Source: CAD feature listing. Evaluate the final solid. Frame: model axes, mm. Face numbers are marked on the shaded views. A direction names the side the tool comes from. Give positions to 0.01 mm unless a question says otherwise; leave off trailing zeros. Order: outer loops, then holes, each group sorted by start corner. A loop starts at its lowest first (then second) coordinate and runs counter-clockwise, first axis right, second up. Notation, with made-up numbers: M 46,32 L 82,32 A22 ccw 82,50 Z; hole C -32.5,82.5 d9. An arc over 180 degrees is marked long. Answer in a Markdown table with one row per item. Add a question column.
(1) Section query B-B, the plane x = -9. Return loops of the section in (y, z), plus the area to 3 significant figures.
(2) Pin query (flat end, axial travel): P1, Ø6.5, axis at x = -16, z = -5.5, coming from the +Y side; P2, Ø2.5, axis at x = -28, z = -14, coming from the +Y side; P3, Ø1.5, axis at x = -34, z = 20.5, coming from the +Y side. Return the tip coordinate at first contact, or that it passes through.
(3) Mould query, pull axis Z, two halves, no side actions, for the marked faces 1, 2, 3 and 4. Classes: pulls with the +Z half, pulls with the -Z half, needs draft (parallel to the pull), parting line crosses it, or undercut.
(4) Section query C-C, the plane z = -16.5. Return loops of the section in (x, y), plus the area to 4 significant figures.
(5) Material intervals for line 1 along X through (y, z) = (26.5, -16); line 2 along X through (y, z) = (27.5, -20); line 3 along X through (y, z) = (19.5, -5), sorted ascending.
(6) Set-up query: the marked faces 5, 6 and 7. Return all of +Z, -Z, +X, -X, +Y, -Y with unobstructed straight access to the full face (end or side cutting, diameter ignored); none if empty.
(7) Section query D-D, the plane z = 13.5. Return loops of the section in (x, y), plus the area to 4 significant figures.
(8) Section query A-A, the plane y = 19.5. Return loops of the section in (x, z).
from build123d import *

# Parameters (mm, degrees)
SKETCH_1_W          = 47.5
SKETCH_1_H          = 60.8
EXTRUDE_1_DEPTH     = 30
SKETCH_2_R          = 1
EXTRUDE_3_DEPTH     = 5
SKETCH_3_W          = 37.5
SKETCH_3_H          = 45.8
CUT_EXTRUDE_1_DEPTH = 27
SKETCH_4_W          = 14
SKETCH_4_H          = 5
CUT_EXTRUDE_2_DEPTH = 8
SKETCH_5_R          = 3
SKETCH_5_W          = 6
SKETCH_5_H          = 6
EXTRUDE_4_DEPTH     = 20.5
SKETCH_6_W          = 5
SKETCH_6_H          = 10.5
EXTRUDE_6_DEPTH     = 25
SKETCH_7_R          = 1
EXTRUDE_7_DEPTH     = 5
SKETCH_12_W         = 5.3
SKETCH_12_H         = 4.5
CUT_EXTRUDE_5_DEPTH = 10
SKETCH_13_W         = 1.5
SKETCH_13_H         = 6
EXTRUDE_8_DEPTH     = 4.5


with BuildPart() as part:
    # 草图1 → 凸台-拉伸1 (new body)
    with BuildSketch(Plane(origin=(0, 0, 0), x_dir=(1, 0, 0), z_dir=(0, 1, 0))):
        with Locations((-26.283333333, -1.583333333)):
            Rectangle(SKETCH_1_W, SKETCH_1_H)
    extrude(amount=EXTRUDE_1_DEPTH)

    # 草图2 → 凸台-拉伸3 (add)
    with BuildSketch(Plane(origin=(0, 30, 0), x_dir=(1, 0, 0), z_dir=(0, 1, 0))):
        with Locations(Location((-22.533333333, 26.316666667, 0), (0, 0, 270))):
            Circle(SKETCH_2_R)
        with Locations(Location((-47.533333333, 26.316666667, 0), (0, 0, 270))):
            Circle(SKETCH_2_R)
        with Locations(Location((-47.533333333, -29.483333333, 0), (0, 0, 270))):
            Circle(SKETCH_2_R)
        with Locations(Location((-5.033333333, -29.483333333, 0), (0, 0, 270))):
            Circle(SKETCH_2_R)
    extrude(amount=EXTRUDE_3_DEPTH)

    # 草图3 → 切除-拉伸1 (cut)
    with BuildSketch(Plane(origin=(0, 30, 0), x_dir=(1, 0, 0), z_dir=(0, 1, 0))):
        with Locations((-26.283333333, -4.083333333)):
            Rectangle(SKETCH_3_W, SKETCH_3_H)
    extrude(amount=-CUT_EXTRUDE_1_DEPTH, mode=Mode.SUBTRACT)

    # 草图4 → 切除-拉伸2 (cut)
    with BuildSketch(Plane(origin=(0, 30, 0), x_dir=(1, 0, 0), z_dir=(0, 1, 0))):
        with Locations((-26.083333333, -29.483333333)):
            Rectangle(SKETCH_4_W, SKETCH_4_H)
    extrude(amount=-CUT_EXTRUDE_2_DEPTH, mode=Mode.SUBTRACT)

    # 草图5 → 凸台-拉伸4 (add)
    with BuildSketch(Plane(origin=(0, 3, 0), x_dir=(1, 0, 0), z_dir=(0, 1, 0))):
        with Locations(Location((-16.083333333, 4.816666667, 0), (0, 0, 270))):
            Circle(SKETCH_5_R)
        with Locations(Location((-36.483333333, 4.816666667, 0), (0, 0, 270))):
            Circle(SKETCH_5_R)
        with Locations((-25.533333333, -23.983333333)):
            Rectangle(SKETCH_5_W, SKETCH_5_H)
    extrude(amount=EXTRUDE_4_DEPTH)

    # 草图6 → 凸台-拉伸6 (add)
    with BuildSketch(Plane(origin=(0, 3, 0), x_dir=(1, 0, 0), z_dir=(0, 1, 0))):
        with Locations((-28.533333333, 13.566666667)):
            Rectangle(SKETCH_6_W, SKETCH_6_H)
    extrude(amount=EXTRUDE_6_DEPTH)

    # 草图7 → 凸台-拉伸7 (add)
    with BuildSketch(Plane(origin=(0, 23.5, 0), x_dir=(1, 0, 0), z_dir=(0, 1, 0))):
        with Locations(Location((-36.483333333, 4.816666667, 0), (0, 0, 270))):
            Circle(SKETCH_7_R)
        with Locations(Location((-16.083333333, 4.816666667, 0), (0, 0, 270))):
            Circle(SKETCH_7_R)
    extrude(amount=EXTRUDE_7_DEPTH)

    # 草图12 → 切除-拉伸5 (cut)
    with BuildSketch(Plane(origin=(0, 0, -28.816666667), x_dir=(-1, 0, 0), z_dir=(0, 0, -1))):
        with Locations((13.183333333, 27.75)):
            Rectangle(SKETCH_12_W, SKETCH_12_H)
    extrude(amount=-CUT_EXTRUDE_5_DEPTH, mode=Mode.SUBTRACT)

    # 草图13 → 凸台-拉伸8 (add)
    with BuildSketch(Plane(origin=(0, 25.5, 0), x_dir=(1, 0, 0), z_dir=(0, 1, 0))):
        with Locations((-13.183333333, 21.816666667)):
            Rectangle(SKETCH_13_W, SKETCH_13_H)
    extrude(amount=EXTRUDE_8_DEPTH)


solid = part.part
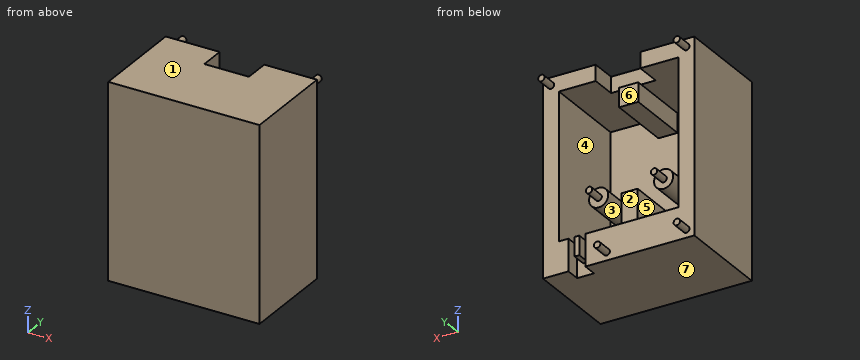
Values follow:
| question | item | result |
|---|---|---|
| 1 | outline | M 0,-28.82 L 30,-28.82 L 30,-18.82 L 3,-18.82 L 3,26.98 L 30,26.98 L 30,31.98 L 0,31.98 Z |
| 1 | area | 587 mm² |
| 2 | P1 | stops at y = 28.5 |
| 2 | P2 | stops at y = 28 |
| 2 | P3 | stops at y = 3 |
| 3 | face 1 | pulls with the +Z half |
| 3 | face 2 | needs draft |
| 3 | face 3 | undercut |
| 3 | face 4 | undercut |
| 4 | outline | M -50.03,0 L -2.53,0 L -2.53,30 L -7.53,30 L -7.53,3 L -26.03,3 L -26.03,28 L -31.03,28 L -31.03,3 L -45.03,3 L -45.03,30 L -50.03,30 Z |
| 4 | area | 537.5 mm² |
| 5 | line 1 | x = -50.03 to -45.03, -31.03 to -26.03, -7.53 to -2.53 |
| 5 | line 2 | x = -50.03 to -15.83, -13.93 to -12.43, -10.53 to -2.53 |
| 5 | line 3 | x = -50.03 to -45.03, -39.48 to -33.49, -19.08 to -13.09, -7.53 to -2.53 |
| 6 | face 5 | +Y |
| 6 | face 6 | +Z, +Y |
| 6 | face 7 | -Z, +X, -X, +Y, -Y |
| 7 | outline | M -50.03,0 L -2.53,0 L -2.53,30 L -7.53,30 L -7.53,3 L -45.03,3 L -45.03,30 L -50.03,30 Z |
| 7 | area | 412.5 mm² |
| 8 | outline | M -50.03,-28.82 L -2.53,-28.82 L -2.53,31.98 L -50.03,31.98 Z; C -36.48,-4.82 d6; C -16.08,-4.82 d6; hole M -45.03,-18.82 L -31.03,-18.82 L -31.03,-8.32 L -26.03,-8.32 L -26.03,-18.82 L -7.53,-18.82 L -7.53,26.98 L -22.53,26.98 L -22.53,20.98 L -28.53,20.98 L -28.53,26.98 L -45.03,26.98 Z |
